Autodesk Inventor part; units mm, degrees
ref_plane "YZ Plane" through (0, 0, 0) normal (1, 0, 0) x (0, 1, 0)
ref_plane "XZ Plane" through (0, 0, 0) normal (0, 1, 0) x (-1, 0, 0)
ref_plane "XY Plane" through (0, 0, 0) normal (0, 0, 1) x (1, 0, 0)
sketch "Szkic1" plane through (0, 0, 0) normal (0, 0, 1) x (1, 0, 0)
  line L0 (-58.8, 0) -> (58.8, 0)
  line L1 (0, -5.1) -> (0, 30.6)
  line L2 (0, 0) -> (42, 0)
  line L3 (42, 0) -> (42, 25.5)
  line L4 (42, 25.5) -> (0, 25.5)
  line L5 (0, 25.5) -> (0, 0)
  circle A0 centre (39.5, 23) radius 1.2
  circle A1 centre (39.5, 3) radius 1.2
  point P0 (0, 25.5)
  point P1 (42, 0)
  dimension "d0" = 25.5
  dimension "d1" = 42
  dimension "d7" = 2.4
  dimension "d8" = 2.4
  dimension "d9" = 2.5
  dimension "d10" = 2.5
  dimension "d11" = 20
  dimension "d12" = 2.5
extrude "Wyciągnięcie proste1" add sketch "Szkic1" along normal blind 2
sketch "Szkic2" plane through (42, 0, 0) normal (1, 0, 0) x (0, 0, -1)
  line L0 (0, 0) -> (0, 25.5)
  line L1 (0, 25.5) -> (-2, 25.5)
  line L2 (-2, 0) -> (-2, 25.5)
  line L3 (0, 0) -> (-2, 0)
  line L4 (0, 25.5) -> (0, 0)
  line L5 (0, 0) -> (-2, 0.7279)
  line L6 (-2, 25.5) -> (-2, 0)
  point P0 (0, 0)
  dimension "d4" = 70
extrude "Wyciągnięcie proste2" cut sketch "Szkic2" against normal blind 90 contours L3 L2 L5
mirror "Odbij1" about plane through (0, 0, 0) normal (1, 0, 0) of "Wyciągnięcie proste1", "Wyciągnięcie proste2"
sketch "Sketch3" plane through (0, 0, 2) normal (0, 0, 1) x (1, 0, 0)
  line L0 (-42, 0.7279) -> (42, 0.7279)
  line L1 (42, 0.7279) -> (42, 25.5)
  line L2 (42, 25.5) -> (-42, 25.5)
  line L3 (-42, 0.7279) -> (-42, 25.5)
  circle A0 centre (-39.5, 23) radius 1.2
  circle A1 centre (-39.5, 3) radius 1.2
  circle A2 centre (39.5, 23) radius 1.2
  circle A3 centre (39.5, 3) radius 1.2
  line L4 (42, 0) -> (42, 25.5)
  line L5 (42, 20.25) -> (32.5, 20.25)
  line L6 (32.5, 20.25) -> (32.5, 5.75)
  line L7 (32.5, 5.75) -> (42, 5.75)
  line L8 (42, 5.75) -> (42, 20.25)
  point P0 (0, 0)
  point P1 (32.5, 13)
  dimension "d13" = 9.5
  dimension "d14" = 14.5
  dimension "d15" = 10
extrude "Extrusion3" cut sketch "Sketch3" against normal blind 10 contours L7 L6 L5 L1
properties part number "góra_robota" material "Tworzywo sztuczne PET"
Model file for the job. Use its own axes, mm. A direction names the side the tool comes from. Coordinates: 2 decimals unless noted, no trailing zeros. Write each loop counter-clockwise with the first axis right and the second up, starting at its lowest first coordinate (ties: lowest second). Pieces come first, ordered by that corner, then holes. Notation, with made-up numbers: (63.25, -14) - (91.25, -14) arc R17 ccw to (91.25, 18) - close; hole circle Ø9 at (54, 52). An arc over 180 degrees is marked (long way). Use a Markdown table: item, result. Add a question column.
Item 1: 3-axis set-ups, long thin cutter, end or side, ignore diameter. For faces 1 (the face through (37, 20.25, 1)), 2 (the face through (-42, 13, 1)): which of +Z, -Z, +X, -X, +Y, -Y reach the whole face in a straight line?
Item 2: Drop flat-ended pins along their axis: pin 1 (4 mm diameter, centred on x = 39.5, y = 3, fed in from -Z); pin 2 (2 mm diameter, centred on x = -39.5, y = 23, fed in from -Z). Give the stop position or say it passes through.
Item 3: Two-plate mould, pull along Y, no slides. Class faces 3 (the face through (42, 23, 1)), 4 (the face through (-40.61, 22.54, 0.99)), 5 (the face through (0.59, 0.36, 0.99)): pulls with the +Y half, pulls with the -Y half, needs draft (parallel to the pull), parting line crosses it, or undercut.
Item 4: Band-saw the part on A-A, the plane x = 39.5. Write the cut outline in (y, z), and give its area (3 significant figures).
Item 5: Band-saw the part on C-C, the plane x = -39.5. Write the cut outline in (y, z).
Item 6: Band-saw the part on B-B, the plane y = 3. Write the cut outline in (x, z).
Item 7: Drill centre lines: line 1 along Y through (x, z) = (39.5, 1.15); line 2 along X through (y, z) = (4, 1); line 3 along X through (y, z) = (22.5, 0.9). Where is each one in solid material? Low to high.
Item 8: Band-saw the part on D-D, the plane z = 1.05. Write the cut outline in (x, y).
A:
| question | item | result |
|---|---|---|
| 1 | face 1 | +Z, -Z, +X |
| 1 | face 2 | +Z, -Z, -X, +Y, -Y |
| 2 | pin 1 | stops at z = 0 |
| 2 | pin 2 | passes through |
| 3 | face 3 | needs draft |
| 3 | face 4 | undercut |
| 3 | face 5 | pulls with the -Y half |
| 4 | outline | (0, 0) - (1.8, 0) - (1.8, 2) - (0.73, 2) - close; (4.2, 0) - (5.75, 0) - (5.75, 2) - (4.2, 2) - close; (20.25, 0) - (21.8, 0) - (21.8, 2) - (20.25, 2) - close; (24.2, 0) - (25.5, 0) - (25.5, 2) - (24.2, 2) - close |
| 4 | area | 11.7 mm² |
| 5 | outline | (0, 0) - (1.8, 0) - (1.8, 2) - (0.73, 2) - close; (4.2, 0) - (21.8, 0) - (21.8, 2) - (4.2, 2) - close; (24.2, 0) - (25.5, 0) - (25.5, 2) - (24.2, 2) - close |
| 6 | outline | (-42, 0) - (-40.7, 0) - (-40.7, 2) - (-42, 2) - close; (-38.3, 0) - (38.3, 0) - (38.3, 2) - (-38.3, 2) - close; (40.7, 0) - (42, 0) - (42, 2) - (40.7, 2) - close |
| 7 | line 1 | y = 0.42 to 1.8, 4.2 to 5.75, 20.25 to 21.8, 24.2 to 25.5 |
| 7 | line 2 | x = -42 to -40.16, -38.84 to 38.84, 40.16 to 42 |
| 7 | line 3 | x = -42 to -40.59, -38.41 to 38.41, 40.59 to 42 |
| 8 | outline | (-42, 0.38) - (42, 0.38) - (42, 5.75) - (32.5, 5.75) - (32.5, 20.25) - (42, 20.25) - (42, 25.5) - (-42, 25.5) - close; hole circle Ø2.4 at (-39.5, 3); hole circle Ø2.4 at (-39.5, 23); hole circle Ø2.4 at (39.5, 3); hole circle Ø2.4 at (39.5, 23) |
